Here's how the part is built. I have some questions about the finished solid (model axes, mm). A direction names the side the tool comes from. Coordinates: 2 decimals unless noted, no trailing zeros. Loops run counter-clockwise (first coordinate to the right, second up) from the corner with the lowest first, then second, coordinate; pieces in that order, holes last. Notation, with made-up numbers: M 34,64 L 41,64 A21 cw 41,82 Z; hole C 81,48 d7. An arc over 180 degrees is marked long. Use CSV: the item, a comma, the result in double quotes. Start each with the question number.
Q1. If we mould it in two halves opening along X, with no side actions, what happens to faces 1 (the flat face through (0, 33, 25)), 2 (the flat face through (-20, 90, 79)), 3 (the cylindrical face through (-3.2, 53.3, 14))? For each: +X half, -X half, draft (parallel to the pull), parting line (faces both ways), or undercut.
Q2. Which directions (+Z, -Z, +X, -X, +Y, -Y) give clear straight access to the entire face, cutting with the end or side of a thin tool? Please do faces 4 (the flat face through (-26, 72, 84)), 5 (the flat face through (-20, 0, 1)), 6 (the flat face through (-14, 72, 84)).
Q3. For pin 1 Ø2.5 at (x, z) = (-20, 68) entering from +Y; pin 2 Ø4.5 at (x, z) = (-4, -15.5) entering from +Y; pin 3 Ø5 at (x, z) = (-7, 87.5) entering from -Y; pin 4 Ø10 at (y, z) = (74.5, 87.5) entering from +X, each with a flat end and sliding along its axis, tell me the tip position at first contact or that it passes through.
Q4. If we section it at B-B (x = -20): State how many separate pieces and enclosed holes the cut face has, and give its area (3 significant figures).
Q5. Please list where these lines run through material, in increasing order: probe 1 along Z at (x, y) = (-35, 53.1); probe 2 along X at (y, z) = (53.65, -15.5); probe 3 along Z at (x, y) = (-20, 87). Write a range as [from, to].
Q6. If we section it at A-A (z = 15.5): Please give me the cut outline in (x, y), and give its area (3 significant figures).
Q7. If we section it at D-D (y = 66): Please give me the cut outline in (x, z), and give its area (3 significant figures).
from build123d import *

# Parameters (mm, degrees)
SKETCH1_W               = 40
SKETCH1_H               = 55
SKETCH1_H_2             = 20
SKETCH1_R               = 2.5
BOSS_EXTRUDE1_DEPTH     = 10
SKETCH3_W               = 40
SKETCH3_H               = 10
BOSS_EXTRUDE2_DEPTH     = 40
SKETCH4_W               = 9
SKETCH4_H               = 3.5
BOSS_EXTRUDE3_DEPTH     = 40
SKETCH5_R               = 1.7
CUT_EXTRUDE1_DEPTH      = 3.5
SKETCH7_W               = 40
SKETCH7_H               = 3.5
BOSS_EXTRUDE4_DEPTH     = 80
SKETCH8_W               = 12
SKETCH8_H               = 40
BOSS_EXTRUDE5_DEPTH     = 35
SKETCH9_W               = 12
SKETCH9_H               = 23
CUT_EXTRUDE2_DEPTH      = 17
SKETCH10_R              = 1.7
CUT_EXTRUDE3_DEPTH      = 1
CUT_EXTRUDE3_DEPTH_BACK = 38.5
FILLET1_R               = 1
FILLET2_R               = 40


with BuildPart() as part:
    # Sketch1 → Boss-Extrude1 (new body)
    with BuildSketch(Plane(origin=(0, 0, 0), x_dir=(0, 0, -1), z_dir=(1, 0, 0))):
        with Locations((0, 27.5)):
            Rectangle(SKETCH1_W, SKETCH1_H)
        with Locations((0, -10)):
            Rectangle(SKETCH1_W, SKETCH1_H_2)
        with Locations((10, -10)):
            Circle(SKETCH1_R, mode=Mode.SUBTRACT)
        with Locations((-10, -10)):
            Circle(SKETCH1_R, mode=Mode.SUBTRACT)
    extrude(amount=BOSS_EXTRUDE1_DEPTH)

    # Sketch3 → Boss-Extrude2 (add)
    with BuildSketch(Plane.ZY):
        with Locations((0, 5)):
            Rectangle(SKETCH3_W, SKETCH3_H)
    extrude(amount=BOSS_EXTRUDE2_DEPTH)

    # Sketch4 → Boss-Extrude3 (add)
    with BuildSketch(Plane.ZY):
        with Locations((-15.5, 53.25)):
            Rectangle(SKETCH4_W, SKETCH4_H)
    boss_extrude3 = extrude(amount=BOSS_EXTRUDE3_DEPTH)

    # Sketch5 → Cut-Extrude1 (cut)
    with BuildSketch(Plane(origin=(0, 55, 0), x_dir=(1, 0, 0), z_dir=(0, 1, 0))):
        with Locations((-35, 15.5)):
            Circle(SKETCH5_R)
        with Locations((-4, 15.5)):
            Circle(SKETCH5_R)
    cut_extrude1 = extrude(amount=-CUT_EXTRUDE1_DEPTH, mode=Mode.SUBTRACT)

    # Mirror2: Boss-Extrude3, Cut-Extrude1 across plane
    add(boss_extrude3.mirror(Plane.XY))
    add(cut_extrude1.mirror(Plane.XY), mode=Mode.SUBTRACT)

    # Sketch7 → Boss-Extrude4 (add)
    with BuildSketch(Plane.XY.offset(20)):
        with Locations((-20, 53.25)):
            Rectangle(SKETCH7_W, SKETCH7_H)
        Polygon((10, 55), (0, 55), (0, 51.5), (0, 25), (10, 25), align=None)
    extrude(amount=BOSS_EXTRUDE4_DEPTH)

    # Sketch8 → Boss-Extrude5 (add)
    with BuildSketch(Plane(origin=(0, 55, 0), x_dir=(1, 0, 0), z_dir=(0, 1, 0))):
        with Locations((-20, -80)):
            Rectangle(SKETCH8_W, SKETCH8_H)
    extrude(amount=BOSS_EXTRUDE5_DEPTH)

    # Sketch9 → Cut-Extrude2 (cut)
    with BuildSketch(Plane(origin=(0, 0, 60), x_dir=(-1, 0, 0), z_dir=(0, 0, -1))):
        with Locations((20, 72.5)):
            Rectangle(SKETCH9_W, SKETCH9_H)
    extrude(amount=-CUT_EXTRUDE2_DEPTH, mode=Mode.SUBTRACT)

    # Sketch10 → Cut-Extrude3 (cut, two sides)
    with BuildSketch(Plane(origin=(0, 90, 0), x_dir=(1, 0, 0), z_dir=(0, 1, 0))) as cut_extrude3_sk:
        with Locations((-20, -68)):
            Circle(SKETCH10_R)
    extrude(amount=CUT_EXTRUDE3_DEPTH, mode=Mode.SUBTRACT)
    extrude(cut_extrude3_sk.sketch, amount=-CUT_EXTRUDE3_DEPTH_BACK, mode=Mode.SUBTRACT)

    # Fillet1
    fillet1_edges = [part.edges().sort_by_distance(p)[0] for p in [
        (-33, 55, 100),
        (-26, 55, 80),
        (-26, 87, 60),
        (-26, 72.5, 100),
        (-14, 55, 80),
        (-14, 72.5, 100),
        (-20, 55, 60),
        (-14, 87, 60),
        (-26, 90, 80),
        (-20, 90, 100),
        (-14, 90, 80),
        (-26, 58, 60),
        (-14, 58, 60),
        (-14, 72.5, 77),
        (-14, 61, 68.5),
        (-20, 84, 77),
        (-14, 84, 68.5),
        (-26, 72.5, 77),
        (-26, 84, 68.5),
        (-20, 61, 77),
        (-26, 61, 68.5),
        (-20, 51.5, 100),
        (0, 38.25, 100),
        (5, 25, 100),
        (10, 40, 100),
        (-2, 55, 100),
        (-40, 53.25, 100),
    ]]
    fillet(fillet1_edges, radius=FILLET1_R)

    # Fillet2
    fillet2_edges = [part.edges().sort_by_distance(p)[0] for p in [
        (5, 25, 20),
    ]]
    fillet(fillet2_edges, radius=FILLET2_R)


solid = part.part
Results below:
1,face 1,"-X half"
1,face 2,"draft"
1,face 3,"undercut"
2,face 4,"+Z, -Z, -X, +Y"
2,face 5,"+Z, -Z, -X, -Y"
2,face 6,"+Z, -Z, +X, +Y"
3,pin 1,"through"
3,pin 2,"y = 55"
3,pin 3,"y = 51.5"
3,pin 4,"x = -14"
4,separate pieces,"5"
4,enclosed holes,"0"
4,area,"1,750 mm^2"
5,probe 1,"[-20, -17.2], [-13.8, -11], [11, 13.8], [17.2, 100]"
5,probe 2,"[-40, -36.7], [-33.3, -5.7], [-2.3, 10]"
5,probe 3,"[60, 66.3], [69.7, 100]"
6,outline,"M -40,0 L 0,0 L 0,-20 L 10,-20 L 10,55 L -2.3,55 L -2.3,51.5 L 0,51.5 L 0,10 L -40,10 Z; M -40,51.5 L -36.7,51.5 L -36.7,55 L -40,55 Z; M -33.3,51.5 L -5.7,51.5 L -5.7,55 L -33.3,55 Z"
6,area,"1,270 mm^2"
7,outline,"M -26,78 A1 ccw -25,77 L -15,77 A1 ccw -14,78 L -14,99 A1 ccw -15,100 L -25,100 A1 ccw -26,99 Z"
7,area,"275 mm^2"
